CAD build for the part. Positions are in the model's coordinates, mm. Face numbers are marked on the shaded views. A direction names the side the tool comes from. Round coordinates to 2 decimals unless told otherwise and drop trailing zeros. Loops run counter-clockwise (first coordinate to the right, second up) from the corner with the lowest first, then second, coordinate; pieces in that order, holes last.
Autodesk Inventor part; units mm, degrees
ref_plane "YZ Plane" through (0, 0, 0) normal (1, 0, 0) x (0, 1, 0)
ref_plane "XZ Plane" through (0, 0, 0) normal (0, 1, 0) x (-1, 0, 0)
ref_plane "XY Plane" through (0, 0, 0) normal (0, 0, 1) x (1, 0, 0)
sketch "Sketch1" plane through (0, 0, 0) normal (0, 0, 1) x (1, 0, 0)
  line L0 (0, 0) -> (7.6, 0)
  line L1 (12, -2.5403) -> (12, -6.4)
  line L2 (12, -6.4) -> (5, -6.4)
  line L3 (5, -6.4) -> (5, -26.4)
  line L4 (5, -26.4) -> (0, -26.4)
  line L5 (0, -26.4) -> (0, 0)
  line L6 (7.6, 0) -> (12, -2.5403)
  dimension "d0" = 24
  dimension "d1" = 10
  dimension "d2" = 6.4
  dimension "d3" = 20
  dimension "d20" = 30
  dimension "d21" = 15.2
revolve "Вращение1" add sketch "Sketch1" angle 360 about axis through (0, -26.4, 0) along (0, 1, 0)
sketch "Sketch2" plane through (0, 0, 0) normal (0, 1, 0) x (1, 0, 0)
  line L0 (0, -9.2376) -> (-8, -4.6188)
  line L1 (-8, -4.6188) -> (-8, 4.6188)
  line L2 (-8, 4.6188) -> (0, 9.2376)
  line L3 (0, 9.2376) -> (8, 4.6188)
  line L4 (8, 4.6188) -> (8, -4.6188)
  line L5 (8, -4.6188) -> (0, -9.2376)
  circle A0 centre (0, 0) radius 12
  point P0 (0, 0)
  point P1 (0, 0)
  dimension "d22" = 16
extrude "Выдавливание1" cut sketch "Sketch2" against normal blind 6.4
thread "Резьба1"
chamfer "Фаска1" distance 0.8333 angle 45 1 edges at (-5, -26.4, 0)
equation "\"d22\" = S_"
equation "\"d23\" = k"
equation "\"d12\" = b"
equation "\"d14\" = 0.0833333 * d"
equation "\"d0\" = 1.5 * S_"
equation "\"d1\" = d1_"
equation "\"d2\" = k"
equation "\"d3\" = L"
equation "\"d21\" = 0.95 * S_"
equation "\"d1_\" = 10"
equation "\"S_\" = 16"
equation "\"k\" = 6.4"
equation "\"e\" = 17.6"
equation "\"L\" = 20"
equation "\"b\" = 18"
equation "\"Grip_Length\" = 2"
properties part number "Болт M10-6g×20(S16) ГОСТ 7798-70" material "Сталь, мягкая"
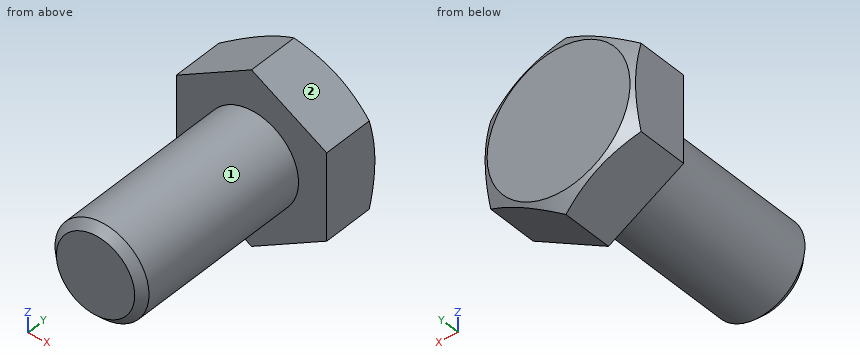
Item 1: Flat gauge pins, fed straight in: P1, Ø1, axis at y = -20, z = 1.5, coming from the +X side; P2, Ø1, axis at y = -19, z = -4.5, coming from the +X side; P3, Ø8, axis at y = -22.5, z = -6, coming from the +X side. Where does each tip first touch, or does it go through?
Verdict:
P1: stops at x = 4.9
P2: stops at x = 3
P3: stops at x = 4.58
Item 2: Cut at B-B (z = 0). List the corners of the cut face in (x, y).
Verdict:
outline: (-8, -6.4) - (-5, -6.4) - (-5, -25.57) - (-4.17, -26.4) - (4.17, -26.4) - (5, -25.57) - (5, -6.4) - (8, -6.4) - (8, -0.23) - (7.6, 0) - (-7.6, 0) - (-8, -0.23) - close
Item 3: Wall check: L1, parallel to Z at x = 0, y = -16; L2, parallel to Y at x = -1, z = 7.5; L3, parallel to Z at x = 3, y = -17.5. Give the ranges that are in metal, low to high.
Verdict:
L1: z = -5 to 5
L2: y = -6.4 to 0
L3: z = -4 to 4
Item 4: 3-axis set-ups, long thin cutter, end or side, ignore diameter. For the marked faces 1 and 2: which of +Z, -Z, +X, -X, +Y, -Y reach the whole face in a straight line?
Verdict:
face 1: -Y
face 2: +Z, +X, +Y, -Y
Item 5: Cut at C-C (y = -22.5). List the corners of the cut face in (x, z), plus the area to 3 significant figures.
Verdict:
outline: circle Ø10 at (0, 0)
area: 78.5 mm2
Item 6: Cut at A-A (y = -1.75). List the corners of the cut face in (x, z).
Verdict:
outline: (-8, -4.62) - (0, -9.24) - (8, -4.62) - (8, 4.62) - (0, 9.24) - (-8, 4.62) - close
